Source: CAD feature listing. Evaluate the final solid. Frame: model axes, mm. Coordinates: 2 decimals unless noted, no trailing zeros. Loops run counter-clockwise (first coordinate to the right, second up) from the corner with the lowest first, then second, coordinate; pieces in that order, holes last. Notation, with made-up numbers: (13.5, 49.25) - (35.5, 49.25) arc R28 cw to (35.5, 88.25) - close; hole circle Ø4 at (-7.75, 21.5). An arc over 180 degrees is marked (long way). Write item = value, one per line. Start each with the question number.
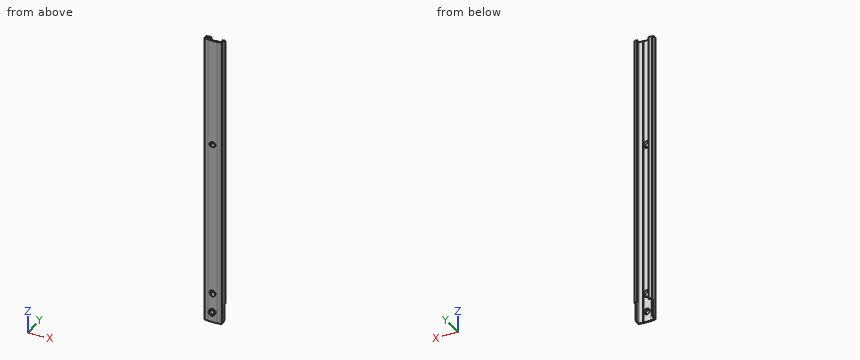
from build123d import *

# Parameters (mm, degrees)
BASE_EXTRU_MINCE_DEPTH            = 330
CONG_1_R                          = 1.5
CONG_2_R                          = 0.5
ENL_V_MAT_EXTRU_1_DEPTH           = 331.295417013
ENL_V_MAT_EXTRU_1_DEPTH_BACK      = 331.295417013
ESQUISSE3_R                       = 3
ENL_V_MAT_EXTRU_4_DEPTH           = 3
BOSS_EXTRU_1_START                = 2
ESQUISSE4_R                       = 3.5
ESQUISSE4_R_2                     = 3
BOSS_EXTRU_1_DEPTH                = 2
CONG_3_R                          = 0.5
ESQUISSE5_R                       = 4.25
BOSS_EXTRU_2_DEPTH                = 1.5
BOSS_EXTRU_2_DRAFT                = -45
BOSS_EXTRU_2_PROFILE_2_DEPTH      = 1.5
BOSS_EXTRU_2_PROFILE_2_DRAFT      = -45
ESQUISSE6_R                       = 4
ENL_V_MAT_EXTRU_6_DEPTH           = 2
ENL_V_MAT_EXTRU_6_DRAFT           = -45
ENL_V_MAT_EXTRU_6_PROFILE_2_DEPTH = 2
ENL_V_MAT_EXTRU_6_PROFILE_2_DRAFT = -45


with BuildPart() as part:
    # Esquisse1 → Base-Extru.-Mince (new body)
    with BuildSketch(Plane.XY):
        Polygon((-6.25, 10), (-9.75, 10), (-9.75, 0.5), (-5, 0.5), (-5, 0), (5, 0), (5, 0.5), (9.75, 0.5), (9.75, 10), (6.25, 10), (6.25, 9), (8.75, 9), (8.75, 1.5), (4, 1.5), (4, 1), (-4, 1), (-4, 1.5), (-8.75, 1.5), (-8.75, 9), (-6.25, 9), align=None)
    extrude(amount=BASE_EXTRU_MINCE_DEPTH)

    # Congé1
    cong_1_edges = [part.edges().sort_by_distance(p)[0] for p in [
        (-9.75, 10, 165),
        (-9.75, 0.5, 165),
        (9.75, 0.5, 165),
        (9.75, 10, 165),
    ]]
    fillet(cong_1_edges, radius=CONG_1_R)

    # Congé2
    cong_2_edges = [part.edges().sort_by_distance(p)[0] for p in [
        (-8.75, 9, 165),
        (-8.75, 1.5, 165),
        (8.75, 1.5, 165),
        (8.75, 9, 165),
    ]]
    fillet(cong_2_edges, radius=CONG_2_R)

    # Esquisse2 → Enlèv. mat.-Extru.1 (cut, two sides: drawn at the far end of the back side and taken through both)
    with BuildSketch(Plane(origin=(0, 0, 0), x_dir=(0, 0, -1), z_dir=(1, 0, 0)).offset(-ENL_V_MAT_EXTRU_1_DEPTH_BACK)):
        with BuildLine():
            Line((-330, 0), (-330, 4.2))
            ThreePointArc((-330, 4.2), (-329.179898987, 6.179898987), (-327.2, 7))
            Line((-327.2, 7), (-327, 7))
            Line((-327, 7), (-327, 10))
            Line((-327, 10), (-332.428830769, 10))
            Line((-332.428830769, 10), (-332.428830769, 0))
            Line((-332.428830769, 0), (-330, 0))
        make_face()
        with BuildLine():
            Line((0.919813001, 11.16366228), (-20, 11.16366228))
            Line((-20, 11.16366228), (-20, 7))
            Line((-20, 7), (-2.8, 7))
            ThreePointArc((-2.8, 7), (-0.820101013, 6.179898987), (0, 4.2))
            Line((0, 4.2), (0, 0))
            Line((0, 0), (0.919813001, 0))
            Line((0.919813001, 0), (0.919813001, 11.16366228))
        make_face()
    extrude(amount=ENL_V_MAT_EXTRU_1_DEPTH + ENL_V_MAT_EXTRU_1_DEPTH_BACK, mode=Mode.SUBTRACT)

    # Esquisse3 → Enlèv. mat.-Extru.4 (cut)
    with BuildSketch(Plane(origin=(0, 0, 0), x_dir=(1, 0, 0), z_dir=(0, 1, 0))):
        with Locations(Location((0, -12, 0), (0, 0, 90))):
            Circle(ESQUISSE3_R)
    extrude(amount=ENL_V_MAT_EXTRU_4_DEPTH, mode=Mode.SUBTRACT)

    # Esquisse4 → Boss.-Extru.1 (add)
    with BuildSketch(Plane.XZ.offset(BOSS_EXTRU_1_START)):
        with Locations(Location((0, 12, 0), (0, 0, 90))):
            Circle(ESQUISSE4_R)
        with Locations(Location((0, 12, 0), (0, 0, 270))):
            Circle(ESQUISSE4_R_2, mode=Mode.SUBTRACT)
    extrude(amount=-BOSS_EXTRU_1_DEPTH)

    # Congé3
    cong_3_edges = [part.edges().sort_by_distance(p)[0] for p in [
        (0, 1, 15),
    ]]
    fillet(cong_3_edges, radius=CONG_3_R)


with BuildPart() as boss_extru_2_tool:
    # Esquisse5 → Boss.-Extru.2 (with draft: the straight prism first)
    with BuildSketch(Plane(origin=(0, 1, 0), x_dir=(-1, 0, 0), z_dir=(0, 1, 0))):
        with Locations((0, 208)):
            Circle(ESQUISSE5_R)
    extrude(amount=-BOSS_EXTRU_2_DEPTH)
    # Boss.-Extru.2: the draft: its side faces are tilted about the plane it starts from
    boss_extru_2_sides = [boss_extru_2_tool.faces().sort_by_distance(p)[0] for p in [
        (4.25, 0.25, 208),
    ]]
    draft(boss_extru_2_sides, Plane(origin=(0, 1, 0), x_dir=(-1, 0, 0), z_dir=(0, 1, 0)), BOSS_EXTRU_2_DRAFT)


with BuildPart() as part_1:
    add(part.part)

    # Boss.-Extru.2: add boss_extru_2_tool
    add(boss_extru_2_tool.part)


with BuildPart() as boss_extru_2_profile_2_tool:
    # Esquisse5 → Boss.-Extru.2 profile 2 (with draft: the straight prism first)
    with BuildSketch(Plane(origin=(0, 1, 0), x_dir=(-1, 0, 0), z_dir=(0, 1, 0))):
        with Locations((0, 34)):
            Circle(ESQUISSE5_R)
    extrude(amount=-BOSS_EXTRU_2_PROFILE_2_DEPTH)
    # Boss.-Extru.2 profile 2: the draft: its side faces are tilted about the plane it starts from
    boss_extru_2_profile_2_sides = [boss_extru_2_profile_2_tool.faces().sort_by_distance(p)[0] for p in [
        (4.25, 0.25, 34),
    ]]
    draft(boss_extru_2_profile_2_sides, Plane(origin=(0, 1, 0), x_dir=(-1, 0, 0), z_dir=(0, 1, 0)), BOSS_EXTRU_2_PROFILE_2_DRAFT)


with BuildPart() as part_2:
    add(part_1.part)

    # Boss.-Extru.2 profile 2: add boss_extru_2_profile_2_tool
    add(boss_extru_2_profile_2_tool.part)


with BuildPart() as enl_v_mat_extru_6_tool:
    # Esquisse6 → Enlèv. mat.-Extru.6 (with draft: the straight prism first)
    with BuildSketch(Plane(origin=(0, 1, 0), x_dir=(-1, 0, 0), z_dir=(0, 1, 0))):
        with Locations((0, 33)):
            Circle(ESQUISSE6_R)
    extrude(amount=-ENL_V_MAT_EXTRU_6_DEPTH)
    # Enlèv. mat.-Extru.6: the draft: its side faces are tilted about the plane it starts from
    enl_v_mat_extru_6_sides = [enl_v_mat_extru_6_tool.faces().sort_by_distance(p)[0] for p in [
        (4, 0, 33),
    ]]
    draft(enl_v_mat_extru_6_sides, Plane(origin=(0, 1, 0), x_dir=(-1, 0, 0), z_dir=(0, 1, 0)), ENL_V_MAT_EXTRU_6_DRAFT)


with BuildPart() as part_3:
    add(part_2.part)

    # Enlèv. mat.-Extru.6: cut by enl_v_mat_extru_6_tool
    add(enl_v_mat_extru_6_tool.part, mode=Mode.SUBTRACT)


with BuildPart() as enl_v_mat_extru_6_profile_2_tool:
    # Esquisse6 → Enlèv. mat.-Extru.6 profile 2 (with draft: the straight prism first)
    with BuildSketch(Plane(origin=(0, 1, 0), x_dir=(-1, 0, 0), z_dir=(0, 1, 0))):
        with Locations((0, 208)):
            Circle(ESQUISSE6_R)
    extrude(amount=-ENL_V_MAT_EXTRU_6_PROFILE_2_DEPTH)
    # Enlèv. mat.-Extru.6 profile 2: the draft: its side faces are tilted about the plane it starts from
    enl_v_mat_extru_6_profile_2_sides = [enl_v_mat_extru_6_profile_2_tool.faces().sort_by_distance(p)[0] for p in [
        (4, 0, 208),
    ]]
    draft(enl_v_mat_extru_6_profile_2_sides, Plane(origin=(0, 1, 0), x_dir=(-1, 0, 0), z_dir=(0, 1, 0)), ENL_V_MAT_EXTRU_6_PROFILE_2_DRAFT)


with BuildPart() as part_4:
    add(part_3.part)

    # Enlèv. mat.-Extru.6 profile 2: cut by enl_v_mat_extru_6_profile_2_tool
    add(enl_v_mat_extru_6_profile_2_tool.part, mode=Mode.SUBTRACT)


solid = part_4.part
Item 1: First-contact query: pin 1 (0.6 mm diameter, centred on x = 7, z = 229.5, fed in from -Y); pin 2 (0.5 mm diameter, centred on x = -9, z = 11.5, fed in from +Y); pin 3 (1.5 mm diameter, centred on x = 8, y = 8.5, fed in from +Z). Flat tips, straight axial feed; report the tip coordinate or a pass-through.
Item 2: Cut plane B-B (z = 217.5). Return the cut outline in (x, y), then the cut area to 3 significant figures.
Item 3: Material intervals for L1, parallel to X at y = -1.3, z = 12; L2, parallel to X at y = 3, z = 285; L3, parallel to Y at x = -5.75, z = 200, sorted ascending. Write a range as [from, to].
Responses:
q1.pin_1 = 0.5
q1.pin_2 = 7
q1.pin_3 = 327
q2.outline = (-9.75, 2) arc R1.5 ccw to (-8.25, 0.5) - (-5, 0.5) - (-5, 0) - (5, 0) - (5, 0.5) - (8.25, 0.5) arc R1.5 ccw to (9.75, 2) - (9.75, 8.5) arc R1.5 ccw to (8.25, 10) - (6.25, 10) - (6.25, 9) - (8.25, 9) arc R0.5 cw to (8.75, 8.5) - (8.75, 2) arc R0.5 cw to (8.25, 1.5) - (4, 1.5) - (4, 1) - (-4, 1) - (-4, 1.5) - (-8.25, 1.5) arc R0.5 cw to (-8.75, 2) - (-8.75, 8.5) arc R0.5 cw to (-8.25, 9) - (-6.25, 9) - (-6.25, 10) - (-8.25, 10) arc R1.5 ccw to (-9.75, 8.5) - close
q2.area = 40.8 mm2
q3.L1 = [-3.5, -3], [3, 3.5]
q3.L2 = [-9.75, -8.75], [8.75, 9.75]
q3.L3 = [0.5, 1.5]
